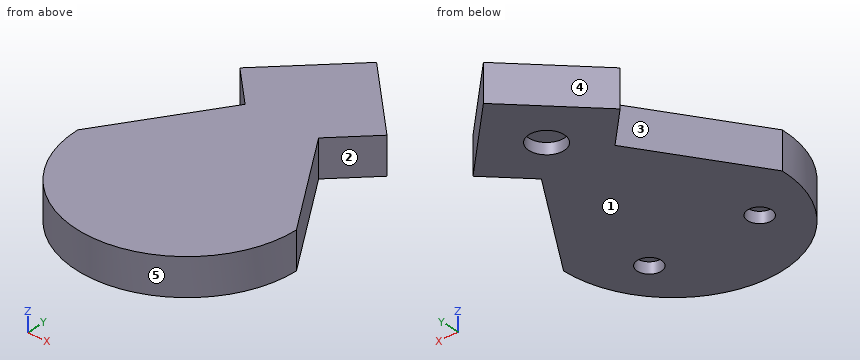
```python
from build123d import *

# Parameters (mm, degrees)
F1_DEPTH = 10
F2_R     = 4.75
F2_R_2   = 3.25
F3_DEPTH = 3


with BuildPart() as f1:
    # F0 (on Top) → F1 (new body)
    with BuildSketch(Plane.XY):
        Polygon((10, -10), (20, 0), (0, 20), (-20, 0), (-10, -10), (0, -20), align=None)
        with BuildLine():
            Line((29.725478, -40), (10, -10))
            Line((10, -10), (0, -20))
            Line((0, -20), (-10, -10))
            Line((-10, -10), (-29.725478, -40))
            ThreePointArc((-29.725478, -40), (0, -69.725478), (29.725478, -40))
        make_face()
    extrude(amount=F1_DEPTH)

    # F2 (on Top) → F3 (cut)
    with BuildSketch(Plane.XY):
        Circle(F2_R)
        with Locations((15, -50)):
            Circle(F2_R_2)
        with Locations((-15, -50)):
            Circle(F2_R_2)
    extrude(amount=F3_DEPTH, mode=Mode.SUBTRACT)


solid = f1.part
```
The listing builds one solid part. Answer for the finished solid, in the listing's coordinates (mm). Face numbers are marked on the shaded views. A direction names the side the tool comes from. Give positions to 0.01 mm unless a question says otherwise; leave off trailing zeros. Order: outer loops, then holes, each group sorted by start corner. A loop starts at its lowest first (then second) coordinate and runs counter-clockwise, first axis right, second up. Notation, with made-up numbers: (-22.75, 80) -> (1.25, 80) arc R18 cw to (1.25, 87) -> close; hole circle Ø8 at (71, 25.25). An arc over 180 degrees is marked (long way). Write each question's results on one line, items separated by ' | '.
Q1. The part is cut by section B-B, the plane z = 5. Give the vertices of the cut face in (x, y).
Checked values:
outline: (-29.73, -40) arc R29.73 ccw to (29.73, -40) -> (10, -10) -> (20, 0) -> (0, 20) -> (-20, 0) -> (-10, -10) -> close
Q2. Each of these flat-tipped pins is pushed along its axis until it touches: P1, Ø2, axis at y = -51.5, z = 2, coming from the -X side; P2, Ø6, axis at x = -15, y = -50, coming from the -Z side; P3, Ø4, axis at y = -6, z = 8, coming from the +X side. Where does it stop, or does it pass through?
Checked values:
P1: stops at x = -27.81 | P2: stops at z = 3 | P3: stops at x = 16
Q3. Determine the mould class of the marked faces 3, 4 and 5 for opening direction Y: pulls with the +Y half, pulls with the -Y half, needs draft (parallel to the pull), parting line crosses it, or undercut.
Checked values:
face 3: undercut | face 4: pulls with the +Y half | face 5: pulls with the -Y half
Q4. Which of the six approach directions +Z, -Z, +X, -X, +Y, -Y give full straight-line access (tool end or side, diameter ignored) to the marked faces 1 and 2?
Checked values:
face 1: -Z, +X, -X, +Y, -Y | face 2: +Z, -Z, +X
Q5. Straight lines are drawn through the part: probe 1 along Y at (x, z) = (0, 2.1); probe 2 along Y at (x, z) = (-15, 1.05); probe 3 along Y at (x, z) = (-18.5, 0.5). For each, find the intervals that lie inside material, in ascending order. Write a range as from..to.
Checked values:
probe 1: y = -69.73..-4.75, 4.75..20 | probe 2: y = -65.66..-53.25, -46.75..-17.6, -5..5 | probe 3: y = -63.27..-22.93, -1.5..1.5
Q6. The part is cut by section C-C, the plane y = -50. Give the vertices of the cut face in (x, z).
Checked values:
outline: (-27.99, 0) -> (-18.25, 0) -> (-18.25, 3) -> (-11.75, 3) -> (-11.75, 0) -> (11.75, 0) -> (11.75, 3) -> (18.25, 3) -> (18.25, 0) -> (27.99, 0) -> (27.99, 10) -> (-27.99, 10) -> close
Q7. The part is cut by section D-D, the plane x = 1. Give the vertices of the cut face in (y, z), and give its area (3 significant figures).
Checked values:
outline: (-69.71, 0) -> (-4.64, 0) -> (-4.64, 3) -> (4.64, 3) -> (4.64, 0) -> (19, 0) -> (19, 10) -> (-69.71, 10) -> close | area: 859 mm^2
Q8. The part is cut by section A-A, the plane x = 15. Give the vertices of the cut face in (y, z).
Checked values:
outline: (-65.66, 0) -> (-53.25, 0) -> (-53.25, 3) -> (-46.75, 3) -> (-46.75, 0) -> (-17.6, 0) -> (-17.6, 10) -> (-65.66, 10) -> close; (-5, 0) -> (5, 0) -> (5, 10) -> (-5, 10) -> close
